Can you work these out from the model? Positions are in its coordinate system, mm. Face numbers are marked on the shaded views. A direction names the side the tool comes from. Coordinates: 2 decimals unless noted, no trailing zeros. Order: outer loops, then holes, each group sorted by start corner. A loop starts at its lowest first (then second) coordinate and runs counter-clockwise, first axis right, second up. Notation, with made-up numbers: (11.25, 10.5) -> (33.25, 10.5) arc R14 ccw to (33.25, 16.5) -> close; hole circle Ø10 at (-30, 42.5). An arc over 180 degrees is marked (long way). Answer as CSV lines item,"result".
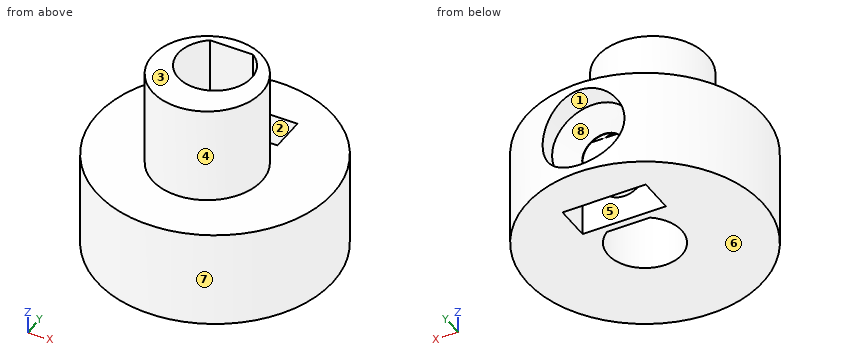
from build123d import *

# Parameters (mm, degrees)
ESQUISSE1_R             = 8.5
BOSS_EXTRU_1_DEPTH      = 7
ESQUISSE2_W             = 6
ESQUISSE2_H             = 2.6
ENL_V_MAT_EXTRU_1_DEPTH = 14.910427743
ESQUISSE7_R             = 2.95
ENL_V_MAT_EXTRU_8_DEPTH = 21.087060672
ESQUISSE9_R             = 3.95
BOSS_EXTRU_2_DEPTH      = 7
ENL_V_MAT_EXTRU_9_DEPTH = 19.45264218


with BuildPart() as part:
    # Esquisse1 → Boss.-Extru.1 (new body)
    with BuildSketch(Plane.XY):
        Circle(ESQUISSE1_R)
    extrude(amount=BOSS_EXTRU_1_DEPTH)

    # Esquisse2 → Enlèv. mat.-Extru.1 (cut, through all)
    with BuildSketch(Plane(origin=(0, 0, 0), x_dir=(-1, 0, 0), z_dir=(0, 0, -1))):
        with Locations((0, 4)):
            Rectangle(ESQUISSE2_W, ESQUISSE2_H)
    extrude(amount=-ENL_V_MAT_EXTRU_1_DEPTH, mode=Mode.SUBTRACT)

    # Enlèv. mat.-Extru.2: read off the stored shape, not the designer's step
    # Enlèv. mat.-Extru.2 outline → Enlèv. mat.-Extru.2 (revolve, cut)
    with BuildSketch(Plane.XY.offset(3.5)):
        Polygon((0, 5.3), (1.554616831, 5.3), (1.498760014, 8.500034923), (0, 8.500034923), align=None)
        Polygon((1.6, 2.7), (0, 2.7), (0, 0.7), (1.56508987, 0.7), align=None)
    revolve(axis=Axis((0, 0, 3.5), (0, 1, 0)), mode=Mode.SUBTRACT)

    # Esquisse7 → Enlèv. mat.-Extru.8 (cut, through all)
    with BuildSketch(Plane(origin=(0, 8.3, 0), x_dir=(1, 0, 0), z_dir=(0, 1, 0))):
        with Locations((0, -3.5)):
            Circle(ESQUISSE7_R)
    extrude(amount=ENL_V_MAT_EXTRU_8_DEPTH, mode=Mode.SUBTRACT)

    # Chanfrein1: read off the stored shape, not the designer's step
    # Chanfrein1 outline → Chanfrein1 (revolve, cut)
    with BuildSketch(Plane.XY.offset(3.5)):
        Polygon((2.95, 6.747748364), (2.95, 8.3), (1.502251636, 8.3), (1.553718474, 5.351466838), align=None)
    revolve(axis=Axis((0, 0, 3.5), (0, 1, 0)), mode=Mode.SUBTRACT)

    # Esquisse9 → Boss.-Extru.2 (add)
    with BuildSketch(Plane.XY.offset(7)):
        with Locations(Location((0, -1, 0), (0, 0, 110.493999506))):
            Circle(ESQUISSE9_R)
    extrude(amount=BOSS_EXTRU_2_DEPTH)

    # Esquisse10 → Enlèv. mat.-Extru.9 (cut, through all)
    with BuildSketch(Plane(origin=(0, 0, 0), x_dir=(-1, 0, 0), z_dir=(0, 0, -1))):
        with BuildLine():
            Line((-1.549193338, 2.15), (1.549193338, 2.15))
            ThreePointArc((1.549193338, 2.15), (0, -2.65), (-1.549193338, 2.15))
        make_face()
    extrude(amount=-ENL_V_MAT_EXTRU_9_DEPTH, mode=Mode.SUBTRACT)


solid = part.part
Q1. We'd pull the mould along X, two halves only. Please class the marked faces 6, 7 and 8: pulls with the +X half, pulls with the -X half, needs draft (parallel to the pull), parting line crosses it, or undercut.
Solution:
face 6,"needs draft"
face 7,"parting line crosses it"
face 8,"undercut"
Q2. Imagine slicing it at B-B (y = 1.5). List the corners of the cut face in (x, z) for me.
Solution:
outline,"(-8.37, 0) -> (-2.18, 0) -> (-2.18, 14) -> (-3.06, 14) -> (-3.06, 7) -> (-8.37, 7) -> close; (2.18, 0) -> (8.37, 0) -> (8.37, 7) -> (3.06, 7) -> (3.06, 14) -> (2.18, 14) -> close"
Q3. Imagine slicing it at D-D (y = -4.5). List the corners of the cut face in (x, z) for me.
Solution:
outline,"(-7.21, 0) -> (7.21, 0) -> (7.21, 7) -> (1.83, 7) -> (1.83, 14) -> (-1.83, 14) -> (-1.83, 7) -> (-7.21, 7) -> close"
Q4. Imagine slicing it at C-C (x = -5.75). List the corners of the cut face in (y, z) for me, and give its area (3 significant figures).
Solution:
outline,"(-6.26, 0) -> (6.26, 0) -> (6.26, 7) -> (-6.26, 7) -> close"
area,"87.6 mm2"
Q5. For P1, Ø3, axis at x = -6.5, y = 4, coming from the +Z side; P2, Ø0.8, axis at y = 4.5, z = 2.5, coming from the -X side; P3, Ø5, axis at y = -1, z = 12, coming from the +X side, each with a flat end and sliding along its axis, tell me the tip position at first contact or that it passes through.
Solution:
P1,"z = 7"
P2,"x = -7.45"
P3,"x = 3.95"
Q6. If I drill on line 1 (Y direction, x = 0, z = 6.5); line 2 (Z direction, x = 0, y = 7.3); line 3 (Y direction, x = 0.75, z = 5.25), over which ranges is the centre line in solid material (lowest first)?
Solution:
line 1,"-8.5 to -2.65, 2.15 to 2.7, 5.3 to 8.5"
line 2,"0 to 0.55, 6.45 to 7"
line 3,"-8.47 to -2.54, 2.15 to 2.7, 5.3 to 5.7"
Q7. Imagine slicing it at A-A (z = 6.75). List the corners of the cut face in (x, y) for me.
Solution:
outline,"circle Ø17 at (0, 0); hole (-3, 2.7) -> (3, 2.7) -> (3, 5.3) -> (-3, 5.3) -> close; hole (-1.55, 2.15) arc R2.65 ccw (long way) to (1.55, 2.15) -> close"
Q8. Which directions (+Z, -Z, +X, -X, +Y, -Y) give clear straight access to the entire face, cutting with the end or side of a thin tool? Please do the marked faces 1, 2, 3, 4 and 5.
Solution:
face 1,"+Y"
face 2,"+Z, -Z"
face 3,"+Z, +X, -X, +Y, -Y"
face 4,"+Z"
face 5,"-Z"
